from build123d import *

# Parameters (mm, degrees)
F3_DEPTH = 13.716
F5_DEPTH = 13.589


with BuildPart() as f1:
    # F0 (on Front) → F1 (revolve)
    with BuildSketch(Plane.XZ):
        Polygon((0, 6.35), (0, 0), (101.6, 0), (101.6, 3.175), (88.9, 3.175), (88.9, 6.35), (82.55, 6.35), (82.55, 7.9375), (50.8, 7.9375), (50.8, 6.2865), (49.53, 6.2865), (49.53, 7.9375), (35.941, 7.9375), (35.941, 6.35), (13.716, 6.35), (13.716, 5.5626), (12.7, 5.5626), (12.7, 6.35), align=None)
    revolve(axis=Axis((121.0162361984, 0, 0), (1, 0, 0)))

    # F2 (on face) → F3 (cut)
    with BuildSketch(Plane(origin=(0, 0, 0), x_dir=(0, -1, 0), z_dir=(-1, 0, 0))):
        with BuildLine():
            Line((0, 6.35), (5.499261314, 3.175))
            ThreePointArc((5.499261314, 3.175), (3.175, 5.499261314), (0, 6.35))
        make_face()
        with BuildLine():
            Line((5.499261314, 3.175), (5.499261314, -3.175))
            ThreePointArc((5.499261314, -3.175), (6.1336289969, -1.6435009364), (6.35, 0))
            ThreePointArc((6.35, 0), (6.1336289969, 1.6435009364), (5.499261314, 3.175))
        make_face()
        with BuildLine():
            Line((5.499261314, -3.175), (0, -6.35))
            ThreePointArc((0, -6.35), (3.175, -5.499261314), (5.499261314, -3.175))
        make_face()
        with BuildLine():
            ThreePointArc((-5.499261314, -3.175), (-3.175, -5.499261314), (0, -6.35))
            Line((0, -6.35), (-5.499261314, -3.175))
        make_face()
        with BuildLine():
            ThreePointArc((-5.499261314, 3.175), (-6.35, 0), (-5.499261314, -3.175))
            Line((-5.499261314, -3.175), (-5.499261314, 3.175))
        make_face()
        with BuildLine():
            ThreePointArc((0, 6.35), (-3.175, 5.499261314), (-5.499261314, 3.175))
            Line((-5.499261314, 3.175), (0, 6.35))
        make_face()
    extrude(amount=-F3_DEPTH, mode=Mode.SUBTRACT)

    # F4 (on face) → F5 (cut, through all)
    with BuildSketch(Plane(origin=(35.941, 0, 0), x_dir=(0, -1, 0), z_dir=(-1, 0, 0))):
        with BuildLine():
            Line((6.7679427578, 4.1471504768), (6.9755090451, -3.7876351213))
            ThreePointArc((6.9755090451, -3.7876351213), (7.6932440913, -1.953945138), (7.9375, 0))
            ThreePointArc((7.9375, 0), (7.6395173895, 2.1544559185), (6.7679427578, 4.1471504768))
        make_face()
        with BuildLine():
            ThreePointArc((6.7679427578, 4.1471504768), (3.7876351213, 6.9755090451), (-0.2075662873, 7.934785598))
            Line((-0.2075662873, 7.934785598), (6.7679427578, 4.1471504768))
        make_face()
        with BuildLine():
            ThreePointArc((-0.2075662873, 7.934785598), (-4.1471504768, 6.7679427578), (-6.9755090451, 3.7876351213))
            Line((-6.9755090451, 3.7876351213), (-0.2075662873, 7.934785598))
        make_face()
        with BuildLine():
            ThreePointArc((-6.9755090451, 3.7876351213), (-7.934785598, -0.2075662873), (-6.7679427578, -4.1471504768))
            Line((-6.7679427578, -4.1471504768), (-6.9755090451, 3.7876351213))
        make_face()
        with BuildLine():
            Line((6.9755090451, -3.7876351213), (0.2075662873, -7.934785598))
            ThreePointArc((0.2075662873, -7.934785598), (4.1471504768, -6.7679427578), (6.9755090451, -3.7876351213))
        make_face()
        with BuildLine():
            Line((0.2075662873, -7.934785598), (-6.7679427578, -4.1471504768))
            ThreePointArc((-6.7679427578, -4.1471504768), (-3.7876351213, -6.9755090451), (0.2075662873, -7.934785598))
        make_face()
    extrude(amount=-F5_DEPTH, mode=Mode.SUBTRACT)


solid = f1.part
Here's how the part is built. I have some questions about the finished solid (model axes, mm). A direction names the side the tool comes from. Round coordinates to 2 decimals unless told otherwise and drop trailing zeros. Loops run counter-clockwise (first coordinate to the right, second up) from the corner with the lowest first, then second, coordinate; pieces in that order, holes last.
1. If I drill on line 1 along X through (y, z) = (5.25, -2.75); line 2 along X through (y, z) = (-2.5, 6); line 3 along X through (y, z) = (-0.5, 4.25), over which ranges is the centre line in solid material (lowest first)?
Answer list:
line 1: x = 0 to 12.7, 13.72 to 88.9
line 2: x = 35.94 to 49.53, 50.8 to 82.55
line 3: x = 0 to 88.9
2. If we section it at C-C on x = 31.5: Write out the boundary of the cut face in (y, z).
Answer list:
outline: circle Ø12.7 at (0, 0)
3. If we section it at B-B on x = 67.5: Write out the boundary of the cut face in (y, z) (1 decimal).
Answer list:
outline: circle Ø15.9 at (0, 0)
4. Which directions (+Z, -Z, +X, -X, +Y, -Y) give clear straight access to the entire face, cutting with the end or side of a thin tool? Please do faces 4 (the face through (12.7, 5, 3)), 5 (the face through (42.64, -3.64, -5.83)), 6 (the face through (49.53, 6, -3)).
Answer list:
face 4: +Z, +Y
face 5: -Z, -X, -Y
face 6: none
5. We'd pull the mould along X, two halves only. Please class faces 1 (the face through (35.941, -3, 6)), 2 (the face through (12.7, -5, -3)), 3 (the face through (95.16, 3.1, -0.69)): +X half, -X half, draft (parallel to the pull), parting line (faces both ways), or undercut.
Answer list:
face 1: -X half
face 2: undercut
face 3: draft
6. For P1, Ø8, axis at y = 5.5, z = 6, coming from the +X side; P2, Ø4, axis at y = 2.5, z = -0.5, coming from the -X side; P3, Ø5, axis at x = 6.5, z = 0.5, coming from the +Y side; P4, Ø6, axis at x = 87.5, z = 0, coming from the -Y side, each with a flat end and sliding along its axis, tell me the tip position at first contact or that it passes through.
Answer list:
P1: stops at x = 88.9
P2: stops at x = 0
P3: stops at y = 5.5
P4: stops at y = -6.35
